Here's how the part is built. I have some questions about the finished solid (model axes, mm). A direction names the side the tool comes from. Round coordinates to 2 decimals unless told otherwise and drop trailing zeros. Write each loop counter-clockwise with the first axis right and the second up, starting at its lowest first coordinate (ties: lowest second). Pieces come first, ordered by that corner, then holes. Notation, with made-up numbers: (14.25, 83) - (47.25, 83) arc R5 ccw to (47.25, 87) - close; hole circle Ø6 at (1.5, -28). An arc over 180 degrees is marked (long way). One line per question, with ' | ' between items. Start each with the question number.
(1) Imagine slicing it at C-C (z = 3). Write out the boundary of the cut face in (x, y).
(2) Imagine slicing it at A-A (y = 3.25). Write out the boundary of the cut face in (x, z), plus the area to 3 significant figures.
(3) For faces 1 (the cylindrical face through (-3.47, 3.75, 3.49)), 2 (the flat face through (-3, 1, 7.5)), 3 (the cylindrical face through (-5.712, 1.32, 3.698)), which set-ups out of +Z, -Z, +X, -X, +Y, -Y let a thin tool reach every point of the face, with its end or its side?
(4) Thinking about a two-plate mould opening in X: for faces 4 (the flat face through (-8.413, 1, 7)), 5 (the flat face through (-5, 4.739, 7)), 6 (the flat face through (-0.913, 1, 7)), 7 (the cylindrical face through (-6.265, -0.24, 11.302)), which applies, pulls with the +X half, pulls with the -X half, needs draft (parallel to the pull), parting line crosses it, or undercut?
(5) Will these pins go through, and if not, where does the flat tip stop? pin 1 (0.8 mm diameter, centred on x = -4.5, z = 3.5, fed in from +Y); pin 2 (3.5 mm diameter, centred on x = -4.66, y = 0.99, fed in from +Z); pin 3 (1.5 mm diameter, centred on x = -3, y = 3, fed in from -Z).
(6) If I drill on L1, parallel to X at y = 1, z = 11.5; L2, parallel to Y at x = -4, z = 7; L3, parallel to X at y = -0.75, z = 8.75, over which ranges is the centre line in solid material (lowest first)?
(7) Imagine slicing it at D-D (y = 1.5). Write out the boundary of the cut face in (x, z), plus the area to 3 significant figures.
(8) Imagine slicing it at B-B (x = -4). Write out the boundary of the cut face in (y, z).
from build123d import *

# Parameters (mm, degrees)
SKETCH1_W                     = 7.5
SKETCH1_H                     = 7.5
BOSS_EXTRUDE1_DEPTH           = 15
HOLE_FOR_TUBING_R             = 1.1
CUT_EXTRUDE1_DEPTH            = 16
F_10_32_HOLE_FOR_LUER_SCREW_R = 2.0193
CUT_EXTRUDE2_DEPTH            = 7.5
F_5_40_SET_SCREW_HOLE_R       = 1.28905
CUT_EXTRUDE3_DEPTH            = 2


with BuildPart() as part:
    # Sketch1 → Boss-Extrude1 (new body)
    with BuildSketch(Plane.XY):
        with Locations((-4.663043478, 0.989130435)):
            Rectangle(SKETCH1_W, SKETCH1_H)
    extrude(amount=BOSS_EXTRUDE1_DEPTH)

    # hole for tubing → Cut-Extrude1 (cut, through all)
    with BuildSketch(Plane(origin=(0, 0, 0), x_dir=(-1, 0, 0), z_dir=(0, 0, -1))):
        with Locations((4.663043478, 0.989130435)):
            Circle(HOLE_FOR_TUBING_R)
    extrude(amount=-CUT_EXTRUDE1_DEPTH, mode=Mode.SUBTRACT)

    # 10-32 hole for luer screw → Cut-Extrude2 (cut)
    with BuildSketch(Plane.XY.offset(15)):
        with Locations((-4.663043478, 0.989130435)):
            Circle(F_10_32_HOLE_FOR_LUER_SCREW_R)
    extrude(amount=-CUT_EXTRUDE2_DEPTH, mode=Mode.SUBTRACT)

    # 5-40 set screw hole → Cut-Extrude3 (cut)
    with BuildSketch(Plane(origin=(0, 4.739130435, 0), x_dir=(1, 0, 0), z_dir=(0, 1, 0))):
        with Locations((-4.663043478, -3)):
            Circle(F_5_40_SET_SCREW_HOLE_R)
    extrude(amount=-CUT_EXTRUDE3_DEPTH, mode=Mode.SUBTRACT)


solid = part.part
Check sheet entries:
1) outline: (-8.41, -2.76) - (-0.91, -2.76) - (-0.91, 4.74) - (-3.37, 4.74) - (-3.37, 2.74) - (-5.95, 2.74) - (-5.95, 4.74) - (-8.41, 4.74) - close; hole circle Ø2.2 at (-4.66, 0.99)
2) outline: (-8.41, 0) - (-0.91, 0) - (-0.91, 15) - (-8.41, 15) - close; hole circle Ø2.58 at (-4.66, 3) | area: 107 mm^2
3) face 1: +Y | face 2: +Z | face 3: +Z, -Z
4) face 4: pulls with the -X half | face 5: needs draft | face 6: pulls with the +X half | face 7: undercut
5) pin 1: y = 2.74 | pin 2: z = 7.5 | pin 3: z = 0
6) L1: -8.41 to -6.68, -2.64 to -0.91 | L2: -2.76 to 0.11, 1.87 to 4.74 | L3: -8.41 to -5.69, -3.64 to -0.91
7) outline: (-8.41, 0) - (-5.64, 0) - (-5.64, 7.5) - (-6.62, 7.5) - (-6.62, 15) - (-8.41, 15) - close; (-3.69, 0) - (-0.91, 0) - (-0.91, 15) - (-2.71, 15) - (-2.71, 7.5) - (-3.69, 7.5) - close | area: 68.6 mm^2
8) outline: (-2.76, 0) - (0.11, 0) - (0.11, 7.5) - (-0.92, 7.5) - (-0.92, 15) - (-2.76, 15) - close; (1.87, 0) - (4.74, 0) - (4.74, 1.89) - (2.74, 1.89) - (2.74, 4.11) - (4.74, 4.11) - (4.74, 15) - (2.9, 15) - (2.9, 7.5) - (1.87, 7.5) - close
